```python
from build123d import *

# Parameters (mm, degrees)
F1_DEPTH    = 6.985
F2_T1_DEPTH = 6.985
F3_R        = 1.27
F4_R        = 1.27


# Not quite as in the source:
# - a fillet or chamfer that OpenCascade refuses, or shapes differently, is made with other operations: its cross-section is extruded or revolved along the edge and cut away or added
# - a feature names something its author has since deleted; it is built from what else it names


with BuildPart() as f1:
    # F0 (on Top) → F1 (new body)
    with BuildSketch(Plane.XY):
        with BuildLine():
            Line((0, 15.6591), (0, 11.0109))
            ThreePointArc((0, 11.0109), (7.785882057, 7.785882057), (11.0109, 0))
            ThreePointArc((11.0109, 0), (10.6357126807, -2.8498306237), (9.5357191185, -5.50545))
            Line((9.5357191185, -5.50545), (13.5611784004, -7.82955))
            Line((13.5611784004, -7.82955), (18.2062211237, 0.2159))
            Line((18.2062211237, 0.2159), (9.2900854465, 15.6591))
            Line((9.2900854465, 15.6591), (0, 15.6591))
        make_face()
        with BuildLine():
            ThreePointArc((-9.5357191185, -5.50545), (-9.5357191185, 5.50545), (0, 11.0109))
            Line((0, 11.0109), (0, 15.6591))
            Line((0, 15.6591), (-9.2900854465, 15.6591))
            Line((-9.2900854465, 15.6591), (-18.2062211237, 0.2159))
            Line((-18.2062211237, 0.2159), (-13.5611784004, -7.82955))
            Line((-13.5611784004, -7.82955), (-9.5357191185, -5.50545))
        make_face()
        with BuildLine():
            Line((13.5611784004, -7.82955), (9.5357191185, -5.50545))
            ThreePointArc((9.5357191185, -5.50545), (0, -11.0109), (-9.5357191185, -5.50545))
            Line((-9.5357191185, -5.50545), (-13.5611784004, -7.82955))
            Line((-13.5611784004, -7.82955), (-8.9161356771, -15.875))
            Line((-8.9161356771, -15.875), (8.9161356771, -15.875))
            Line((8.9161356771, -15.875), (13.5611784004, -7.82955))
        make_face()
        with BuildLine():
            Line((-9.2900854465, 15.6591), (0, 15.6591))
            Line((0, 15.6591), (0, 20.7391))
            ThreePointArc((0, 20.7391), (-2.8498306237, 21.1142873193), (-5.50545, 22.2142808815))
            Line((-5.50545, 22.2142808815), (-9.2900854465, 15.6591))
        make_face()
        with BuildLine():
            Line((0, 20.7391), (0, 15.6591))
            Line((0, 15.6591), (9.2900854465, 15.6591))
            Line((9.2900854465, 15.6591), (5.50545, 22.2142808815))
            ThreePointArc((5.50545, 22.2142808815), (2.8498306237, 21.1142873193), (0, 20.7391))
        make_face()
        with BuildLine():
            Line((18.2062211237, 0.2159), (13.5611784004, -7.82955))
            Line((13.5611784004, -7.82955), (17.9605874516, -10.36955))
            ThreePointArc((17.9605874516, -10.36955), (19.7104245132, -8.089117943), (21.9908565702, -6.3392808815))
            Line((21.9908565702, -6.3392808815), (18.2062211237, 0.2159))
        make_face()
        with BuildLine():
            Line((17.9605874516, -10.36955), (13.5611784004, -7.82955))
            Line((13.5611784004, -7.82955), (8.9161356771, -15.875))
            Line((8.9161356771, -15.875), (16.4854065702, -15.875))
            ThreePointArc((16.4854065702, -15.875), (16.8605938895, -13.0251693763), (17.9605874516, -10.36955))
        make_face()
        with BuildLine():
            Line((-8.9161356771, -15.875), (-13.5611784004, -7.82955))
            Line((-13.5611784004, -7.82955), (-17.9605874516, -10.36955))
            ThreePointArc((-17.9605874516, -10.36955), (-16.8605938895, -13.0251693763), (-16.4854065702, -15.875))
            Line((-16.4854065702, -15.875), (-8.9161356771, -15.875))
        make_face()
        with BuildLine():
            Line((-17.9605874516, -10.36955), (-13.5611784004, -7.82955))
            Line((-13.5611784004, -7.82955), (-18.2062211237, 0.2159))
            Line((-18.2062211237, 0.2159), (-21.9908565702, -6.3392808815))
            ThreePointArc((-21.9908565702, -6.3392808815), (-19.7104245132, -8.089117943), (-17.9605874516, -10.36955))
        make_face()
        with BuildLine():
            Line((5.50545, 22.2142808815), (9.2900854465, 15.6591))
            Line((9.2900854465, 15.6591), (11.6907231639, 15.6591))
            Line((11.6907231639, 15.6591), (18.9159874322, 37.8961768904))
            Line((18.9159874322, 37.8961768904), (0, 51.6394462192))
            Line((0, 51.6394462192), (-18.9159874322, 37.8961768904))
            Line((-18.9159874322, 37.8961768904), (-11.6907231639, 15.6591))
            Line((-11.6907231639, 15.6591), (-9.2900854465, 15.6591))
            Line((-9.2900854465, 15.6591), (-5.50545, 22.2142808815))
            ThreePointArc((-5.50545, 22.2142808815), (-5.50545, 41.2857191185), (11.0109, 31.75))
            ThreePointArc((11.0109, 31.75), (9.5357191185, 26.24455), (5.50545, 22.2142808815))
        make_face()
        with BuildLine():
            Line((16.4854065702, -15.875), (8.9161356771, -15.875))
            Line((8.9161356771, -15.875), (7.7158168185, -17.9540132485))
            Line((7.7158168185, -17.9540132485), (23.3610581773, -35.3298140992))
            Line((23.3610581773, -35.3298140992), (44.7210722631, -25.8197231096))
            Line((44.7210722631, -25.8197231096), (42.2770456095, -2.5663627912))
            Line((42.2770456095, -2.5663627912), (19.4065399823, 2.2949132485))
            Line((19.4065399823, 2.2949132485), (18.2062211237, 0.2159))
            Line((18.2062211237, 0.2159), (21.9908565702, -6.3392808815))
            ThreePointArc((21.9908565702, -6.3392808815), (33.0017565702, -6.3392808815), (38.5072065702, -15.875))
            ThreePointArc((38.5072065702, -15.875), (27.4963065702, -26.8859), (16.4854065702, -15.875))
        make_face()
        with BuildLine():
            Line((-21.9908565702, -6.3392808815), (-18.2062211237, 0.2159))
            Line((-18.2062211237, 0.2159), (-19.4065399823, 2.2949132485))
            Line((-19.4065399823, 2.2949132485), (-42.2770456095, -2.5663627912))
            Line((-42.2770456095, -2.5663627912), (-44.7210722631, -25.8197231096))
            Line((-44.7210722631, -25.8197231096), (-23.3610581773, -35.3298140992))
            Line((-23.3610581773, -35.3298140992), (-7.7158168185, -17.9540132485))
            Line((-7.7158168185, -17.9540132485), (-8.9161356771, -15.875))
            Line((-8.9161356771, -15.875), (-16.4854065702, -15.875))
            ThreePointArc((-16.4854065702, -15.875), (-37.0320256887, -21.38045), (-21.9908565702, -6.3392808815))
        make_face()
    extrude(amount=F1_DEPTH)

    # F2: fillet of radius 5.08 on 6 edges, made by hand

    # F2_s2 → F2_t1 (join)
    with BuildSketch(Plane.XY):
        with BuildLine():
            ThreePointArc((-11.9396642154, 11.0698949536), (-11.2665307911, 13.3347353028), (-11.6907231639, 15.6591))
            Line((-11.6907231639, 15.6591), (-9.2900854465, 15.6591))
            Line((-9.2900854465, 15.6591), (-11.9396642154, 11.0698949536))
        make_face()
        with BuildLine():
            ThreePointArc((-15.5566423547, 4.8051050464), (-17.1814849205, 3.0897342262), (-19.4065399823, 2.2949132485))
            Line((-19.4065399823, 2.2949132485), (-18.2062211237, 0.2159))
            Line((-18.2062211237, 0.2159), (-15.5566423547, 4.8051050464))
        make_face()
        with BuildLine():
            ThreePointArc((-7.7158168185, -17.9540132485), (-5.9149541295, -16.424469529), (-3.6169781393, -15.875))
            Line((-3.6169781393, -15.875), (-8.9161356771, -15.875))
            Line((-8.9161356771, -15.875), (-7.7158168185, -17.9540132485))
        make_face()
        with BuildLine():
            ThreePointArc((3.6169781393, -15.875), (5.9149541295, -16.424469529), (7.7158168185, -17.9540132485))
            Line((7.7158168185, -17.9540132485), (8.9161356771, -15.875))
            Line((8.9161356771, -15.875), (3.6169781393, -15.875))
        make_face()
        with BuildLine():
            ThreePointArc((19.4065399823, 2.2949132485), (17.1814849205, 3.0897342262), (15.5566423547, 4.8051050464))
            Line((15.5566423547, 4.8051050464), (18.2062211237, 0.2159))
            Line((18.2062211237, 0.2159), (19.4065399823, 2.2949132485))
        make_face()
        with BuildLine():
            ThreePointArc((11.9396642154, 11.0698949536), (11.2665307911, 13.3347353028), (11.6907231639, 15.6591))
            Line((11.6907231639, 15.6591), (9.2900854465, 15.6591))
            Line((9.2900854465, 15.6591), (11.9396642154, 11.0698949536))
        make_face()
    extrude(amount=F2_T1_DEPTH)

    # F3
    f3_edges = [f1.edges().sort_by_distance(p)[0] for p in [
        (9.457994, 44.767812, 6.985),
        (15.303355, 26.777638, 6.985),
        (13.748153, 7.9375, 6.985),
        (11.266531, 13.334735, 6.985),
        (17.181485, 3.089734, 6.985),
        (30.841793, -0.135725, 6.985),
        (43.499059, -14.193043, 6.985),
        (34.041065, -30.574769, 6.985),
        (15.538437, -26.641914, 6.985),
        (0, -15.875, 6.985),
        (-5.914954, -16.42447, 6.985),
        (-15.538437, -26.641914, 6.985),
        (-34.041065, -30.574769, 6.985),
        (-43.499059, -14.193043, 6.985),
        (-30.841793, -0.135725, 6.985),
        (-17.181485, 3.089734, 6.985),
        (-13.748153, 7.9375, 6.985),
        (-11.266531, 13.334735, 6.985),
        (-15.303355, 26.777638, 6.985),
        (-9.457994, 44.767812, 6.985),
        (5.914954, -16.42447, 6.985),
    ]]
    fillet(f3_edges, radius=F3_R)

    # F4
    f4_edges = [f1.edges().sort_by_distance(p)[0] for p in [
        (43.499059, -14.193043, 0),
        (34.041065, -30.574769, 0),
        (15.538437, -26.641914, 0),
        (30.841793, -0.135725, 0),
        (15.303355, 26.777638, 0),
        (9.457994, 44.767812, 0),
        (-9.457994, 44.767812, 0),
        (-15.303355, 26.777638, 0),
        (-13.748153, 7.9375, 0),
        (-30.841793, -0.135725, 0),
        (-34.041065, -30.574769, 0),
        (-15.538437, -26.641914, 0),
        (0, -15.875, 0),
        (13.748153, 7.9375, 0),
        (11.266531, 13.334735, 0),
        (-11.266531, 13.334735, 0),
        (17.181485, 3.089734, 0),
        (-17.181485, 3.089734, 0),
        (5.914954, -16.42447, 0),
        (-5.914954, -16.42447, 0),
    ]]
    fillet(f4_edges, radius=F4_R)


solid = f1.part
```
Check sheet for the modelled part. Datum: model origin and axes. Units: mm. A direction names the side the tool comes from. Round coordinates to 2 decimals unless told otherwise and drop trailing zeros. Order: outer loops, then holes, each group sorted by start corner. A loop starts at its lowest first (then second) coordinate and runs counter-clockwise, first axis right, second up. Notation, with made-up numbers: (54.25, 28) -> (96.25, 28) arc R34 cw to (96.25, 62) -> close; hole circle Ø6 at (22, 58). An arc over 180 degrees is marked (long way). One line per item, written item: value. Start each with the question number.
Q1. Cross-section at A-A (z = 2.5). Record the boundary of the cut face in (x, y) (3 decimals), and give its area (3 significant figures).
Q2. Set-up check for faces 1 (the face through (-14.9, 26.7, 6.6)), 2 (the face through (-13.46, 7.71, 0.38)), 3 (the face through (-5.945, -16.44, 3.461)), 4 (the face through (13.39, 7.79, 0.36)), 5 (the face through (17.21, 3.07, 3.46)): record each of +Z, -Z, +X, -X, +Y, -Y from which the full face is reachable in a straight line by a thin tool's end or side.
Q3. Cross-section at B-B (x = 1.5). Give the number of separate pieces and of enclosed holes in the cut face, and give its area (3 significant figures).
Q4. Thickness scan on line 1 (X direction, y = -26, z = 2.5); line 2 (X direction, y = -13, z = 5); line 3 (Y direction, x = 2.5, z = 1). Record the ranges inside material, lowest first.
Q5. Gauge pin test, flat ends, axial feed: pin 1 Ø1.5 at (x, z) = (12.5, 4) entering from -Y; pin 2 Ø2 at (x, z) = (1.5, 4) entering from -Y (3 decimals); pin 3 Ø2 at (y, z) = (-17, 1.5) entering from +X; pin 4 Ø12 at (x, y) = (-28.5, 37) entering from -Z. Record the tip position at first contact, or that the pin passes through.
Q6. Mould release check, pull along X, two halves, no side actions. Record for faces 6 (the face through (14.99, 27.05, 0.36)), 7 (the face through (-14.89, 26.74, 0.36)), 8 (the face through (-15.71, -26.26, 0.36)), 9 (the face through (-15.648, -26.764, 3.461)): pulls with the +X half, pulls with the -X half, needs draft (parallel to the pull), parting line crosses it, or undercut.
Completed:
1. outline: (-44.721, -25.82) -> (-23.361, -35.33) -> (-7.716, -17.954) arc R5.08 cw to (-3.617, -15.875) -> (3.617, -15.875) arc R5.08 cw to (7.716, -17.954) -> (23.361, -35.33) -> (44.721, -25.82) -> (42.277, -2.566) -> (19.407, 2.295) arc R5.08 cw to (15.557, 4.805) -> (11.94, 11.07) arc R5.08 cw to (11.691, 15.659) -> (18.916, 37.896) -> (0, 51.639) -> (-18.916, 37.896) -> (-11.691, 15.659) arc R5.08 cw to (-11.94, 11.07) -> (-15.557, 4.805) arc R5.08 cw to (-19.407, 2.295) -> (-42.277, -2.566) -> close; hole circle Ø22.022 at (-27.496, -15.875); hole circle Ø22.022 at (0, 0); hole circle Ø22.022 at (0, 31.75); hole circle Ø22.022 at (27.496, -15.875)
1. area: 2,180 mm²
2. face 1: +Z, -X
2. face 2: -Z, -X
2. face 3: +Z, -Z, -Y
2. face 4: -Z, +X
2. face 5: +Z, -Z, +X
3. separate pieces: 3
3. enclosed holes: 0
3. area: 158 mm²
4. line 1: x = -44.32 to -31.82, -23.17 to -14.96, 14.96 to 23.17, 31.82 to 44.32
4. line 2: x = -43.37 to -38.13, -16.87 to 16.87, 38.13 to 43.37
4. line 3: y = -15.85 to -10.72, 10.72 to 21.03, 42.47 to 49.79
5. pin 1: stops at y = -24.1
5. pin 2: stops at y = -15.875
5. pin 3: stops at x = 43.9
5. pin 4: passes through
6. face 6: pulls with the +X half
6. face 7: pulls with the -X half
6. face 8: undercut
6. face 9: undercut
